The listing builds one solid part. Answer for the finished solid, in the listing's coordinates (mm). A direction names the side the tool comes from. Coordinates: 2 decimals unless noted, no trailing zeros. Loops run counter-clockwise (first coordinate to the right, second up) from the corner with the lowest first, then second, coordinate; pieces in that order, holes last. Notation, with made-up numbers: M -38,56 L 1,56 A18 cw 1,78 Z; hole C 80.25,53.5 d6. An arc over 180 degrees is marked long. Answer in a Markdown table with one row per item. Add a question column.
from build123d import *

# Parameters (mm, degrees)
SKETCH_W          = 140
SKETCH_H          = 25
SKETCH_R          = 1.7
PAD_DEPTH         = 11
SKETCH001_W       = 121
SKETCH001_H       = 18
POCKET_DEPTH      = 11.001
POCKET_DEPTH_BACK = 11.001
SKETCH002_W       = 4
SKETCH002_H       = 2
SKETCH002_H_2     = 3.5
PAD001_DEPTH      = 11


with BuildPart() as part:
    # Sketch → Pad (new body, symmetric)
    with BuildSketch(Plane.XZ):
        with Locations((65, 7.5)):
            Rectangle(SKETCH_W, SKETCH_H)
        Circle(SKETCH_R, mode=Mode.SUBTRACT)
    extrude(amount=PAD_DEPTH, both=True)

    # Sketch001 → Pocket (cut, two sides)
    with BuildSketch(Plane.XZ) as pocket_sk:
        with Locations((70.5, 4)):
            Rectangle(SKETCH001_W, SKETCH001_H)
    extrude(amount=-POCKET_DEPTH, mode=Mode.SUBTRACT)
    extrude(pocket_sk.sketch, amount=POCKET_DEPTH_BACK, mode=Mode.SUBTRACT)

    # Sketch002 → Pad001 (join, symmetric)
    with BuildSketch(Plane.XZ):
        with Locations((23.239084, 12)):
            Rectangle(SKETCH002_W, SKETCH002_H)
        with Locations((40.239084, 11.25)):
            Rectangle(SKETCH002_W, SKETCH002_H_2)
    extrude(amount=PAD001_DEPTH, both=True)


solid = part.part
(1) For faces 1 (the face through (16, 0, 13)), 2 (the face through (135, 0, 7)), determine the directions among +Z, -Z, +X, -X, +Y, -Y from which every point of the face is accessible in a straight line to the end or side of a thin tool.
(2) Straight lines are drawn through the part: line 1 (X direction, y = -3.5, z = 10.25); line 2 (X direction, y = -0.25, z = 4.75); line 3 (Z direction, x = 0, y = -5). For each, find the intervals that lie inside material, in ascending order.
(3) A cutting plane is placed at B-B (z = 0). Give the vertices of the cut face in (x, y).
(4) The mould has two halves that part along Z. Classify faces 3 (the face through (2, 0, -5)), 4 (the face through (-0.37, 0.15, -1.66)), 5 (the face through (64, 0, 20)), 6 (the face through (42.239, 0, 11)): released by +Z, released by -Z, zero draft, split by the parting line, or undercut.
(5) A cutting plane is placed at D-D (x = 48.5). Give the vertices of the cut face in (y, z).
(6) A cutting plane is placed at C-C (y = 9.5). Give the vertices of the cut face in (x, z), plus the area to 3 significant figures.
(7) A cutting plane is placed at A-A (x = 0). Give the vertices of the cut face in (y, z).
(8) Each of these flat-tipped pins is pushed along its axis until it touches: pin 1 (6.5 mm diameter, centred on x = 98, y = -1, fed in from -Z); pin 2 (3 mm diameter, centred on x = 23.5, y = -3, fed in from -Z); pin 3 (2 mm diameter, centred on x = 41, y = 3, fed in from -Z). Where does it stop, or does it pass through?
Solved:
| question | item | result |
|---|---|---|
| 1 | face 1 | -Z, +Y, -Y |
| 1 | face 2 | +Z, -Z, +X, +Y, -Y |
| 2 | line 1 | x = -5 to 10, 38.24 to 42.24, 131 to 135 |
| 2 | line 2 | x = -5 to 10, 131 to 135 |
| 2 | line 3 | z = -5 to -1.7, 1.7 to 20 |
| 3 | outline | M -5,-11 L -1.7,-11 L -1.7,11 L -5,11 Z; M 1.7,-11 L 10,-11 L 10,11 L 1.7,11 Z; M 131,-11 L 135,-11 L 135,11 L 131,11 Z |
| 4 | face 3 | released by -Z |
| 4 | face 4 | undercut |
| 4 | face 5 | released by +Z |
| 4 | face 6 | zero draft |
| 5 | outline | M -11,13 L 11,13 L 11,20 L -11,20 Z |
| 6 | outline | M -5,-5 L 10,-5 L 10,13 L 21.24,13 L 21.24,11 L 25.24,11 L 25.24,13 L 38.24,13 L 38.24,9.5 L 42.24,9.5 L 42.24,13 L 131,13 L 131,-5 L 135,-5 L 135,20 L -5,20 Z; hole C 0,0 d3.4 |
| 6 | area | 1,330 mm² |
| 7 | outline | M -11,-5 L 11,-5 L 11,-1.7 L -11,-1.7 Z; M -11,1.7 L 11,1.7 L 11,20 L -11,20 Z |
| 8 | pin 1 | stops at z = 13 |
| 8 | pin 2 | stops at z = 11 |
| 8 | pin 3 | stops at z = 9.5 |
